The model under review builds one solid part; all positions refer to its coordinate system, in mm. Round coordinates to 2 decimals unless told otherwise and drop trailing zeros. Write each loop counter-clockwise with the first axis right and the second up, starting at its lowest first coordinate (ties: lowest second). Pieces come first, ordered by that corner, then holes. Notation, with made-up numbers: M 50.5,-25.75 L 55.5,-25.75 A15 cw 55.5,-14.75 Z; hole C 80,41.25 d9. An arc over 180 degrees is marked long. Write item = value, one per line. Start each with the question number.
Item 1: Take a section at A-A, the plane y = 0. Give the boundary of the cut face in (x, z).
Item 2: For pin 1 Ø5 at (y, z) = (-11.5, 6) entering from -X; pin 2 Ø3 at (y, z) = (4, 1.5) entering from -X; pin 3 Ø1 at (y, z) = (-5, 6.5) entering from +X; pin 4 Ø2.5 at (x, y) = (0, 0) entering from -Z, all flat-tipped, find the tip position at first contact; note any pin that passes through.
Item 3: To check wall thickness, follow line 1 along X through (y, z) = (-0.5, 5); line 2 along Y through (x, z) = (6, 2.75); line 3 along Y through (x, z) = (8.5, 5.75). State the ranges of each line that lie inside material, in increasing order.
Item 4: Take a section at C-C, the plane z = 7.25. Give the boundary of the cut face in (x, y).
Item 5: The part is to be moulded in two halves that separate along Y. For faces 1 (the cylindrical face through (6.271, -10.986, 4.563)), 2 (the flat face through (-4, 0, 0)), 3 (the cylindrical face through (-13.887, -10.648, 5.451)), say which applies: +Y half, -Y half, draft (parallel to the pull), parting line (faces both ways), or undercut.
from build123d import *

# Parameters (mm, degrees)
F0_R           = 17.5
F1_DEPTH       = 9
F2_D           = 3
F2_CSINK_D     = 6.72
F2_CSINK_ANGLE = 90
F3_D           = 2.5
F4_R           = 2


with BuildPart() as f1:
    # F0 (on Top) → F1 (new body)
    with BuildSketch(Plane.XY):
        Circle(F0_R)
    extrude(amount=F1_DEPTH)

    # F2 (through all)
    with Locations(Plane(origin=(0, 0, 0), x_dir=(1, 0, 0), z_dir=(0, 0, -1))):
        with Locations((0, 0)):
            CounterSinkHole(F2_D / 2, F2_CSINK_D / 2, counter_sink_angle=F2_CSINK_ANGLE)

    # F3 (through all)
    with Locations(Plane(origin=(0, 0, 0), x_dir=(1, 0, 0), z_dir=(0, 0, -1))):
        with Locations((6, 12.2062498704), (-6, 12.2062498704)):
            Hole(F3_D / 2)

    # F4
    f4_edges = [f1.edges().sort_by_distance(p)[0] for p in [
        (-17.5, 0, 0),
    ]]
    fillet(f4_edges, radius=F4_R)


solid = f1.part
Response values:
q1.outline = M -17.5,2 A2 ccw -15.5,0 L -3.36,0 L -1.5,1.86 L -1.5,9 L -17.5,9 Z; M 1.5,1.86 L 3.36,0 L 15.5,0 A2 ccw 17.5,2 L 17.5,9 L 1.5,9 Z
q2.pin_1 = -15.01
q2.pin_2 = -17.31
q2.pin_3 = 16.91
q2.pin_4 = through
q3.line_1 = -17.49 to -1.41, 1.41 to 17.49
q3.line_2 = -16.44 to -13.46, -10.96 to 16.44
q3.line_3 = -15.3 to 15.3
q4.outline = C 0,0 d35; hole C -6,-12.21 d2.5; hole C 0,0 d3; hole C 6,-12.21 d2.5
q5.face_1 = undercut
q5.face_2 = draft
q5.face_3 = parting line
